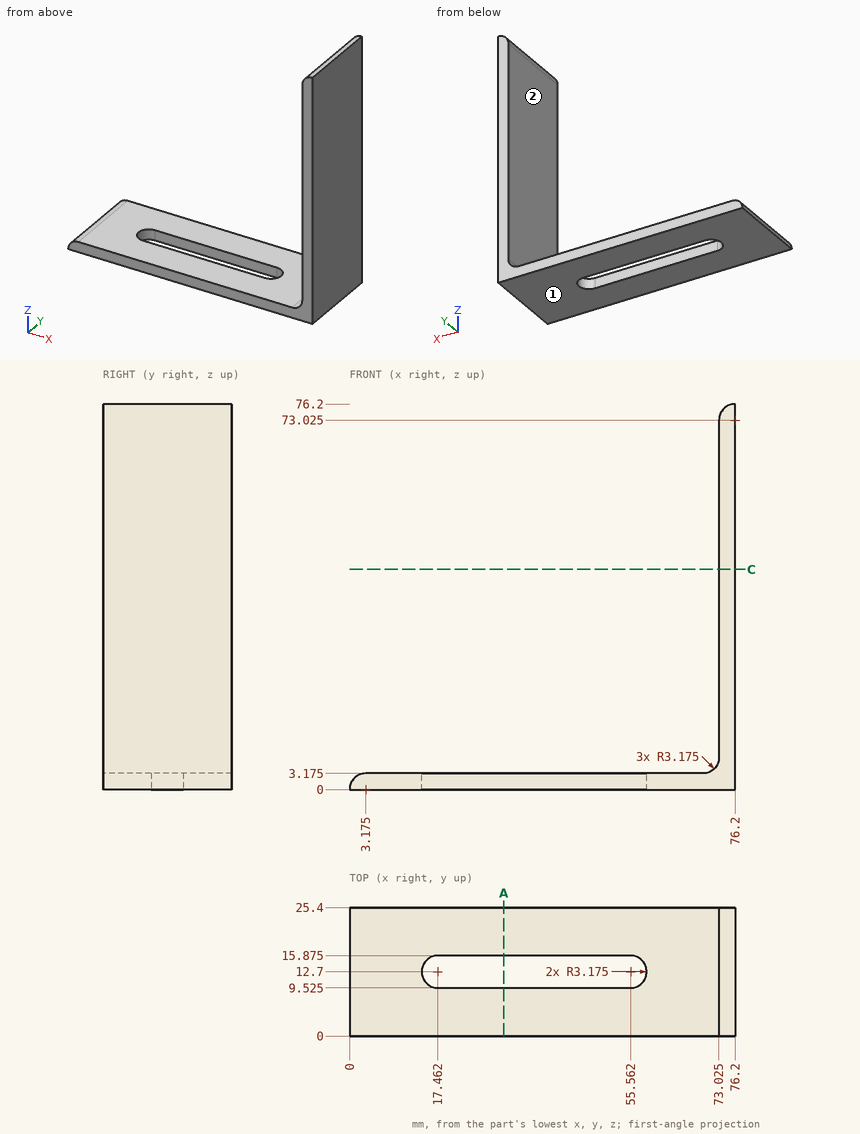
Geometry: see drawing. Coordinates: mm, zero at the bounding-box minimum. A direction names the side the tool comes from. Coordinates: 2 decimals unless noted, no trailing zeros. Write each loop counter-clockwise with the first axis right and the second up, starting at its lowest first coordinate (ties: lowest second). Pieces come first, ordered by that corner, then holes.
1) Pin query (flat end, axial travel): pin 1 Ø7.5 at (y, z) = (12, 44.5) entering from -X (1 decimal); pin 2 Ø3 at (x, y) = (36, 12) entering from +Z; pin 3 Ø3 at (x, y) = (62.5, 22.5) entering from +Z (1 decimal); pin 4 Ø1 at (x, z) = (42, 1.5) entering from -Y. Return the tip coordinate at first contact, or that it passes through.
2) Material intervals for line 1 along Z through (x, y) = (22.5, 23.75) (1 decimal); line 2 along X through (y, z) = (17.75, 65) (1 decimal); line 3 along Z through (x, y) = (72, 9.75) (1 decimal), sorted ascending.
3) Section C-C on z = 43.5. Output: boundary loops of the cut face in (x, y) (1 decimal).
4) Set-up query: the marked faces 1 and 2. Return all of +Z, -Z, +X, -X, +Y, -Y with unobstructed straight access to the full face (end or side cutting, diameter ignored); none if empty.
5) Section A-A on x = 30.5. Output: boundary loops of the cut face in (y, z) (1 decimal).
Check result:
1. pin 1: stops at x = 73
1. pin 2: passes through
1. pin 3: stops at z = 3.2
1. pin 4: stops at y = 0
2. line 1: z = 0 to 3.2
2. line 2: x = 73 to 76.2
2. line 3: z = 0 to 4
3. outline: (73, 0) - (76.2, 0) - (76.2, 25.4) - (73, 25.4) - close
4. face 1: -Z, +X, -X, +Y, -Y
4. face 2: +Z, -X, +Y, -Y
5. outline: (0, 0) - (9.5, 0) - (9.5, 3.2) - (0, 3.2) - close; (15.9, 0) - (25.4, 0) - (25.4, 3.2) - (15.9, 3.2) - close
